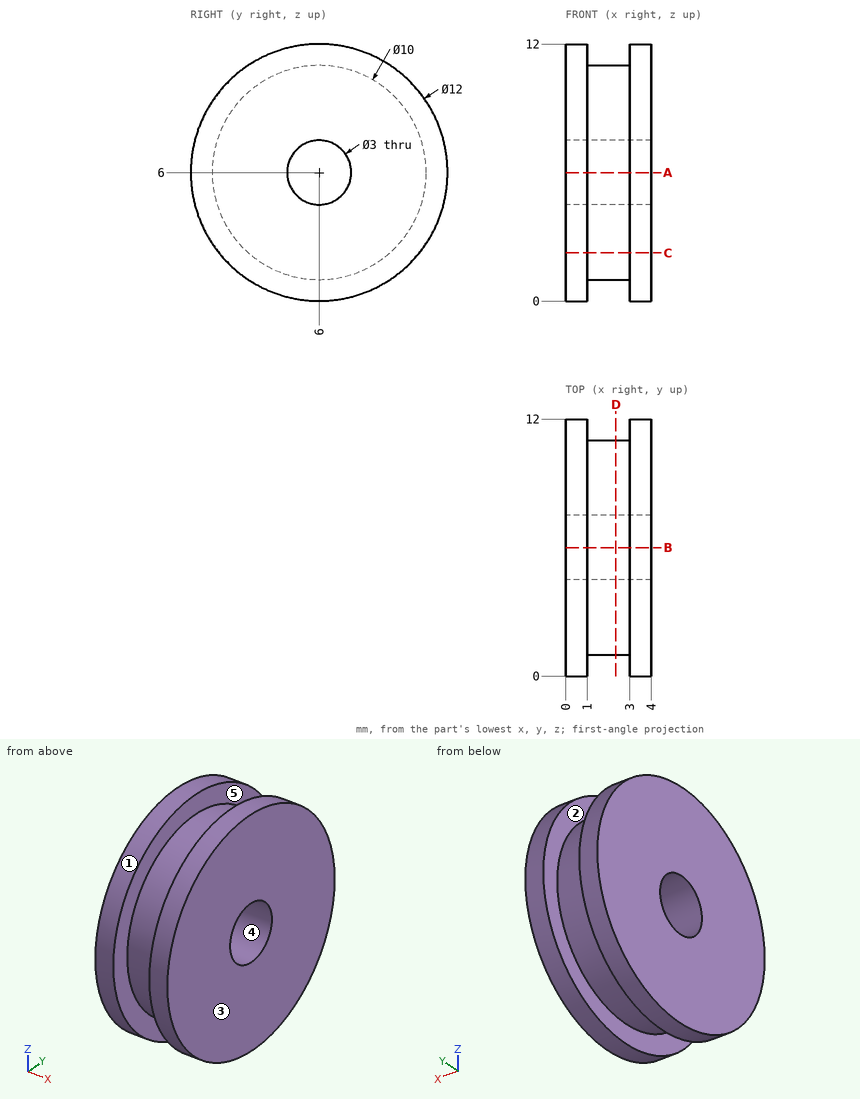
For this review, use the dimensioned drawing (mm, ordinates from the lowest corner) and the shaded views. A direction names the side the tool comes from. Give positions to 0.01 mm unless a question says otherwise; leave off trailing zeros. Loops run counter-clockwise (first coordinate to the right, second up) from the corner with the lowest first, then second, coordinate; pieces in that order, holes last.
Item 1: Take a section at A-A, the plane z = 6. State the section outline as (x, y) points.
Item 2: Take a section at D-D, the plane x = 2.35. State the section outline as (y, z) points.
Item 3: Take a section at C-C, the plane z = 2.25. State the section outline as (x, y) points, and give its area (3 significant figures).
Item 4: For line 1 along X through (y, z) = (4.75, 0.5); line 2 along Z through (x, y) = (1.55, 6); line 3 along Y through (x, z) = (2, 7.25), list the stretches that pass through material, from the lowest coordinate up.
Item 5: Draft analysis for pull direction X (two halves, no side actions). For the marked faces 3, 4 and 5, state which applies: +X half, -X half, draft (parallel to the pull), parting line (faces both ways), or undercut.
Item 6: Tool access review of the marked faces 1 and 2: name each direction out of +Z, -Z, +X, -X, +Y, -Y from which nothing blocks a thin tool from reaching the whole face with its end or side.
Calculated:
1. outline: (0, 0) - (1, 0) - (1, 1) - (3, 1) - (3, 0) - (4, 0) - (4, 4.5) - (0, 4.5) - close; (0, 7.5) - (4, 7.5) - (4, 12) - (3, 12) - (3, 11) - (1, 11) - (1, 12) - (0, 12) - close
2. outline: circle Ø10 at (6, 6); hole circle Ø3 at (6, 6)
3. outline: (0, 1.32) - (1, 1.32) - (1, 2.69) - (3, 2.69) - (3, 1.32) - (4, 1.32) - (4, 10.68) - (3, 10.68) - (3, 9.31) - (1, 9.31) - (1, 10.68) - (0, 10.68) - close
3. area: 32.0 mm2
4. line 1: x = 0 to 1, 3 to 4
4. line 2: z = 1 to 4.5, 7.5 to 11
4. line 3: y = 1.16 to 5.17, 6.83 to 10.84
5. face 3: +X half
5. face 4: draft
5. face 5: undercut
6. face 1: +X, -X
6. face 2: none
